```python
from build123d import *

# Parameters (mm, degrees)
Y_KSEKLIK_EKSTR_ZYON1_DEPTH = 100


with BuildPart() as part:
    # Model → Yükseklik-Ekstrüzyon1 (new body)
    with BuildSketch(Plane.XY):
        with BuildLine():
            Line((-27.777647726, 94.502128478), (-26.508618135, 90.184772354))
            ThreePointArc((-26.508618135, 90.184772354), (-14.704839714, 92.842704016), (-2.657433276, 93.962428919))
            Line((-2.657433276, 93.962428919), (-2.784650827, 98.460630304))
            ThreePointArc((-2.784650827, 98.460630304), (-15.408794806, 97.287301549), (-27.777647726, 94.502128478))
        make_face()
    extrude(amount=Y_KSEKLIK_EKSTR_ZYON1_DEPTH)


with BuildPart() as body_2:
    # Ayır1: the piece on the far side of the plane
    add(part.part)
    split(bisect_by=Plane.XY.offset(50), keep=Keep.BOTTOM)


with BuildPart() as part_1:
    add(part.part)

    # Ayır1
    split(bisect_by=Plane.XY.offset(50), keep=Keep.TOP)


solid = part_1.part
```
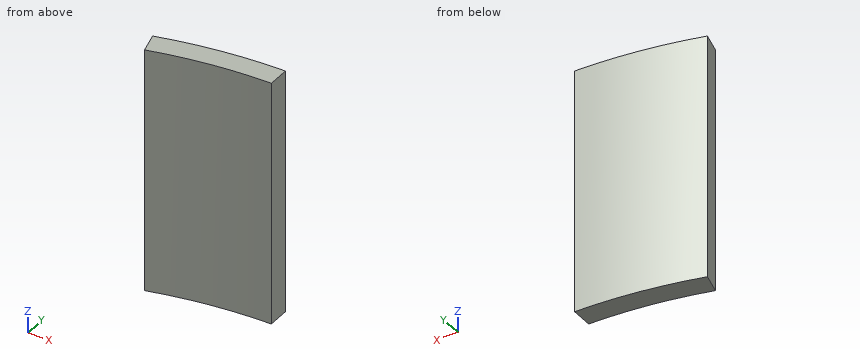
Read the model definition and answer for the solid it produces. Units are mm, in the model's axes. Give positions to 0.01 mm unless a question says otherwise; leave off trailing zeros. Write each loop counter-clockwise with the first axis right and the second up, starting at its lowest first coordinate (ties: lowest second). Pieces come first, ordered by that corner, then holes. Notation, with made-up numbers: (-7, 51.5) -> (50, 51.5) arc R22 ccw to (50, 81.5) -> close; hole circle Ø3 at (-28, 64). An arc over 180 degrees is marked (long way). Answer as a JSON object with one key per item and string values.
1) Section B-B on z = 83 is taken. Write down the section's boundary in (x, y).
Findings below:
{"outline": "(-27.78, 94.5) -> (-26.51, 90.18) arc R94 cw to (-2.66, 93.96) -> (-2.78, 98.46) arc R98.5 ccw to start"}
2) Straight lines are drawn through the part: probe 1 along Y at (x, z) = (-11.5, 63); probe 2 along Y at (x, z) = (-9, 65). For each, find the intervals that lie inside material, in ascending order. Write a range as from..to.
Findings below:
{"probe 1": "y = 93.29..97.83", "probe 2": "y = 93.57..98.09"}
3) Flat-ended cylindrical pins translate along their axes: pin 1 Ø2 at (y, z) = (93.5, 75.5) entering from +X; pin 2 Ø4 at (x, z) = (-22, 90.5) entering from +Y; pin 3 Ø5 at (x, z) = (-11.5, 59.5) entering from +Y; pin 4 Ø10 at (x, z) = (-8.5, 82.5) entering from -Y. Find the tip coordinate at first contact, or state that the pin passes through.
Findings below:
{"pin 1": "stops at x = -2.66", "pin 2": "stops at y = 96.45", "pin 3": "stops at y = 98.09", "pin 4": "stops at y = 93.03"}
4) Section A-A on y = 97.5 is taken. Write down the section's boundary in (x, z).
Findings below:
{"outline": "(-14, 50) -> (-2.76, 50) -> (-2.76, 100) -> (-14, 100) -> close"}
